Check sheet for the modelled part. Datum: model origin and axes. Units: mm. A direction names the side the tool comes from. Give positions to 0.01 mm unless a question says otherwise; leave off trailing zeros. Order: outer loops, then holes, each group sorted by start corner. A loop starts at its lowest first (then second) coordinate and runs counter-clockwise, first axis right, second up.
Autodesk Inventor part; units mm, degrees
ref_plane "YZ Plane" through (0, 0, 0) normal (1, 0, 0) x (0, 1, 0)
ref_plane "XZ Plane" through (0, 0, 0) normal (0, 1, 0) x (-1, 0, 0)
ref_plane "XY Plane" through (0, 0, 0) normal (0, 0, 1) x (1, 0, 0)
ref_plane "Work Plane1" through (-10, 22.6373, -244.9923) normal (-1, 0, 0) x (0, -1, 0)
sketch "Sketch1" plane through (-10, 22.6373, -244.9923) normal (-1, 0, 0) x (0, -1, 0)
  line L0 (26.6373, -5.0077) -> (32.6373, -5.0077) construction
  line L1 (32.6373, -5.0077) -> (32.6373, 244.9923) construction
  line L2 (26.6373, 244.9923) -> (32.6373, 244.9923) construction
  line L3 (26.6373, -5.0077) -> (26.6373, 244.9923) construction
  line L4 (12.6373, -5.0077) -> (18.6373, -5.0077) construction
  line L5 (18.6373, -5.0077) -> (18.6373, 244.9923) construction
  line L6 (12.6373, 244.9923) -> (18.6373, 244.9923) construction
  line L7 (12.6373, -5.0077) -> (12.6373, 244.9923) construction
  line L8 (12.6373, 223.4144) -> (32.6373, 223.4144) construction
  line L9 (32.6373, 223.4144) -> (32.6373, 263.4144) construction
  line L10 (32.6373, 263.4144) -> (12.6373, 263.4144) construction
  line L11 (12.6373, 263.4144) -> (12.6373, 223.4144) construction
  line L12 (12.6373, 263.4144) -> (32.6373, 263.4144) construction
  line L13 (32.6373, 263.4144) -> (32.6373, 223.4144) construction
  line L14 (32.6373, 223.4144) -> (12.6373, 223.4144) construction
  line L15 (12.6373, 223.4144) -> (12.6373, 263.4144) construction
  line L16 (12.6373, 263.4144) -> (32.6373, 263.4144)
  line L17 (32.6373, 263.4144) -> (32.6373, 223.4144)
  line L18 (32.6373, 223.4144) -> (12.6373, 223.4144)
  line L19 (12.6373, 223.4144) -> (12.6373, 263.4144)
  circle A0 centre (22.6373, 258.4144) radius 1.4
  circle A1 centre (22.6373, 251.4144) radius 1.4
  circle A2 centre (22.6373, 244.4144) radius 1.4
  circle A3 centre (22.6373, 237.4144) radius 1.4
  circle A4 centre (22.6373, 230.4144) radius 1.4
  circle A5 centre (22.6373, 223.4144) radius 1.4
  point P0 (22.6373, 244.9923)
  dimension "d0" = 40
  dimension "d1" = 20
  dimension "d2" = 2.8
  dimension "d3" = 5
  dimension "d4" = 10
  dimension "d7" = 7
extrude "Extrusion1" add sketch "Sketch1" along normal blind 6 contours L16 L17 L18 A5 L19 | A5 L18 picked at (22.1842, 223.5261)
sketch "Sketch2" plane through (-10, 10, 18.4222) normal (0, 1, 0) x (1, 0, 0)
  line L0 (0, 0) -> (0, 40)
  line L1 (0, 40) -> (-6, 40)
  line L2 (-6, 0) -> (-6, 40)
  line L3 (0, 0) -> (-6, 0)
  line L4 (-6, 40) -> (-6, 0)
  line L5 (-6, 0) -> (78, 0)
  line L6 (78, 0) -> (78, -6)
  line L7 (78, -6) -> (-6, -6)
  line L8 (-6, -6) -> (-6, 0)
  line L9 (36, 0) -> (44.5, 0)
  line L10 (44.5, 0) -> (44.5, 14.0376)
  line L11 (44.5, 14.0376) -> (36, 14.0376)
  line L12 (36, 14.0376) -> (36, 0)
  line L13 (78, 0) -> (69.5, 0)
  line L14 (69.5, 0) -> (69.5, 14.0376)
  line L15 (69.5, 14.0376) -> (78, 14.0376)
  line L16 (78, 14.0376) -> (78, 0)
  point P0 (10, 18.4222)
  dimension "d14" = 84
  dimension "d15" = 6
  dimension "d16" = 8.5
  dimension "d17" = 36
  dimension "d18" = 8.5
extrude "Extrusion2" add sketch "Sketch2" against normal up to surface (20 mm away) contours L5 L6 L7 L8 L3 | L12 L11 L10 L5 | L14 L15 L16 L5
chamfer "Chamfer1" distance 2 angle 45 4 edges at (-10, 0, 18.4222) (26, 0, 18.4222) (59.5, 0, 18.4222) (34.5, 0, 18.4222)
sketch "Sketch3" plane through (34.5, 10, 4.3845) normal (0, 0, -1) x (-1, 0, 0)
  circle A0 centre (7.15, -8.3308) radius 5.85
  circle A1 centre (-27.35, -10) radius 5.85
  circle A2 centre (-27.35, -10) radius 2.45
  circle A3 centre (7.15, -8.3308) radius 4.1
  point P0 (34.5, -10)
  dimension "d26" = 4.9
extrude "Extrusion3" [suppressed]
properties part number "Neje_Endrole_Adapter"
1) Section check B-B, the plane y = -7.25. Record the cut outline in (x, z), then the cut area to 3 significant figures.
Recorded:
outline: (-16, -21.58) - (-10, -21.58) - (-10, 16.42) - (-8, 18.42) - (24, 18.42) - (26, 16.42) - (26, 4.38) - (34.5, 4.38) - (34.5, 16.42) - (36.5, 18.42) - (57.5, 18.42) - (59.5, 16.42) - (59.5, 4.38) - (68, 4.38) - (68, 24.42) - (-16, 24.42) - close
area: 991 mm2
2) Section check D-D, the plane x = 38. Record the cut outline in (y, z).
Recorded:
outline: (-10, 18.42) - (10, 18.42) - (10, 24.42) - (-10, 24.42) - close
3) Section check A-A, the plane z = 9. Record the cut outline in (x, y), then the cut area to 3 significant figures.
Recorded:
outline: (-16, -10) - (-10, -10) - (-10, 10) - (-16, 10) - close; (26, -10) - (34.5, -10) - (34.5, 10) - (26, 10) - close; (59.5, -10) - (68, -10) - (68, 10) - (59.5, 10) - close
area: 460 mm2
4) Set-up check for faces 1 (the face through (-12.96, 0.3, 7.79)), 2 (the face through (-12.96, -0.75, -1.76)), 3 (the face through (35.49, 0.14, 17.41)): record each of +Z, -Z, +X, -X, +Y, -Y from which the full face is reachable in a straight line by a thin tool's end or side.
Recorded:
face 1: -X
face 2: +X, -X
face 3: -Z, +Y, -Y
5) Material ranges on L1, parallel to X at y = -6, z = 11; L2, parallel to Z at x = -13.7, y = 0; L3, parallel to X at y = 7.5, z = 18, recorded low to high.
Recorded:
L1: x = -16 to -10, 26 to 34.5, 59.5 to 68
L2: z = -21.58 to -15.98, -13.18 to -8.98, -6.18 to -1.98, 0.82 to 5.02, 7.82 to 12.02, 14.82 to 24.42
L3: x = -16 to -8.42, 24.42 to 36.08, 57.92 to 68
6) Depth check by flat-ended pin: pin 1 Ø3.5 at (y, z) = (0, -14.58) entering from +X; pin 2 Ø2 at (y, z) = (0, 13.42) entering from -X; pin 3 Ø9.5 at (x, y) = (31.5, 0.5) entering from -Z; pin 4 Ø2 at (y, z) = (0, -7.58) entering from -X. Enter the tip coordinate at first touch or a pass-through.
Recorded:
pin 1: stops at x = -10
pin 2: stops at x = 26
pin 3: stops at z = 4.38
pin 4: passes through
7) Draft check along X on faces 4 (the face through (68, 0, 14)), 5 (the face through (58.486, -0.14, 17.436)), 6 (the face through (64, 0, 4.385)). Enter one of: +X half, -X half, draft (parallel to the pull), parting line (faces both ways), or undercut.
Recorded:
face 4: +X half
face 5: undercut
face 6: draft
8) Section check C-C, the plane y = 0. State how many separate pieces and enclosed holes the cut face has, then the cut area to 3 significant figures.
Recorded:
separate pieces: 6
enclosed holes: 0
area: 907 mm2
